The listing builds one solid part. Answer for the finished solid, in the listing's coordinates (mm). A direction names the side the tool comes from. Give positions to 0.01 mm unless a question says otherwise; leave off trailing zeros. Write each loop counter-clockwise with the first axis right and the second up, starting at its lowest first coordinate (ties: lowest second). Pieces come first, ordered by that corner, then holes. Notation, with made-up numbers: (-16.75, 8.25) - (-3.75, 8.25) arc R34 ccw to (-3.75, 39.25) - close; hole circle Ø9 at (59.5, -20.75). An arc over 180 degrees is marked (long way). Answer as CSV lines item,"result". Start each with the question number.
(1) Each of these flat-tipped pins is pushed along its axis until it touches: pin 1 Ø1 at (y, z) = (-11, 109.5) entering from -X; pin 2 Ø6 at (x, z) = (157.5, -88.5) entering from +Y; pin 3 Ø12 at (y, z) = (-24, -87.5) entering from +X. Where does it stop, or does it pass through?
(2) Straight lines are drawn through the part: probe 1 along Z at (x, y) = (0, -1); probe 2 along Z at (x, y) = (0, -17); probe 3 along Y at (x, z) = (89, -113). For each, find the intervals that lie inside material, in ascending order.
(3) For faces 4 (the face through (-177.4, -19.8, 55.9)), 5 (the face through (-3, -40, 3)), determine the directions among +Z, -Z, +X, -X, +Y, -Y from which every point of the face is accessible in a straight line to the end or side of a thin tool.
(4) Find section B-B (x = -32.5). Write down the section's boundary in (y, z), then the cut area to 3 significant figures.
(5) Find section A-A (z = 0). Write down the section's boundary in (x, y), then the cut area to 3 significant figures.
(6) For a pull along X with two mould halves and no side action, classify faces 1 (the face through (190.764, -19.72, 60.075)), 2 (the face through (147, 0, -132)), 3 (the face through (3, -35, 3)) as pulls with the +X half, pulls with the -X half, needs draft (parallel to the pull), parting line crosses it, or undercut.
(7) Find section C-C (y = -10.5). Write down the section's boundary in (x, z).
from build123d import *

# Parameters (mm, degrees)
F0_R     = 200
F1_DEPTH = 40
F2_R     = 196
F4_DEPTH = 5
F5_R     = 186
F6_DEPTH = 30


with BuildPart() as f1:
    # F0 (on Front) → F1 (new body)
    with BuildSketch(Plane.XZ):
        Circle(F0_R)
    extrude(amount=F1_DEPTH)

    # F2 (on face) → F4 (cut)
    with BuildSketch(Plane(origin=(0, 0, 0), x_dir=(-1, 0, 0), z_dir=(0, 1, 0))):
        Circle(F2_R)
    extrude(amount=-F4_DEPTH, mode=Mode.SUBTRACT)

    # F5 (on face) → F6 (cut)
    with BuildSketch(Plane(origin=(0, -5, 0), x_dir=(-1, 0, 0), z_dir=(0, 1, 0))):
        Circle(F5_R)
    extrude(amount=-F6_DEPTH, mode=Mode.SUBTRACT)


solid = f1.part
Result set:
1,pin 1,"x = -167.69"
1,pin 2,"y = -35"
1,pin 3,"x = 182.64"
2,probe 1,"-200 to -196, 196 to 200"
2,probe 2,"-200 to -186, 186 to 200"
2,probe 3,"-40 to -35"
3,face 4,"+Y"
3,face 5,"+Z, -Z, +X, -X, -Y"
4,outline,"(-40, -197.34) - (0, -197.34) - (0, -193.29) - (-5, -193.29) - (-5, -183.14) - (-35, -183.14) - (-35, 183.14) - (-5, 183.14) - (-5, 193.29) - (0, 193.29) - (0, 197.34) - (-40, 197.34) - close"
4,area,"2,870 mm^2"
5,outline,"(-200, -40) - (200, -40) - (200, 0) - (196, 0) - (196, -5) - (186, -5) - (186, -35) - (-186, -35) - (-186, -5) - (-196, -5) - (-196, 0) - (-200, 0) - close"
5,area,"2,880 mm^2"
6,face 1,"parting line crosses it"
6,face 2,"needs draft"
6,face 3,"undercut"
7,outline,"circle Ø400 at (0, 0); hole circle Ø372 at (0, 0)"
